The model under review builds one solid part; all positions refer to its coordinate system, in mm. Round coordinates to 2 decimals unless told otherwise and drop trailing zeros. Order: outer loops, then holes, each group sorted by start corner. A loop starts at its lowest first (then second) coordinate and runs counter-clockwise, first axis right, second up. Notation, with made-up numbers: M -39.5,27 L 6.5,27 A16 cw 6.5,41 Z; hole C -3,-35 d7. An arc over 180 degrees is marked long. Answer as a JSON object with one key per item and string values. Group by question number.
1) Consider section B-B, the plane z = 1.8. Count the separate pieces of the cut face and the enclosed holes in it, then the cut area to 3 significant figures.
2) Consider section A-A, the plane x = -129. Write out the cut boundary in (y, z) (3 decimals).
3) To check wall thickness, follow line 1 (X direction, y = 49.5, z = 0.5); line 2 (Y direction, x = -39.5, z = 2.95); line 3 (X direction, y = -125, z = 2.65). State the ranges of each line that lie inside material, in increasing order.
4) Insertion check: pin 1 Ø1.6 at (x, z) = (-99.5, 1) entering from +Y; pin 2 Ø1 at (x, z) = (209, 0.5) entering from -Y; pin 3 Ø7.5 at (x, y) = (-333.55, 0) entering from -Z. Each pin has a flat end and moves straight along its axis. Give the tip position at first contact, or say it passes through.
```python
from build123d import *

# Parameters (mm, degrees)
MASTER_SKETCH_W         = 635.3556
MASTER_SKETCH_H         = 498.348
BOSS_EXTRUDE1_DEPTH     = 3.175
SKETCH2_W               = 31.75
SKETCH2_H               = 498.348
BOSS_EXTRUDE2_DEPTH     = 3.175
M6_CLEARANCE_HOLE1_D    = 6.6
SKETCH5_W               = 2.286
SKETCH5_H               = 69.85
CUT_EXTRUDE1_DEPTH      = 430.182420788
LPATTERN1_COUNT         = 5
LPATTERN1_PITCH         = 98.8568
SKETCH6_W               = 254
SKETCH6_H               = 3.175
CUT_EXTRUDE2_DEPTH      = 430.182420788
SKETCH7_W               = 254
SKETCH7_H               = 2.286
CUT_EXTRUDE3_DEPTH      = 430.182420788
LPATTERN2_COUNT         = 4
LPATTERN2_PITCH         = 98.8568
MIRROR4_COPY_1_SKETCH_W = 254
MIRROR4_COPY_1_SKETCH_H = 2.286
MIRROR4_COPY_1_DEPTH    = 430.182420788
MIRROR4_COPY_2_SKETCH_W = 254
MIRROR4_COPY_2_SKETCH_H = 2.286
MIRROR4_COPY_2_DEPTH    = 430.182420788
MIRROR4_COPY_3_SKETCH_W = 254
MIRROR4_COPY_3_SKETCH_H = 2.286
MIRROR4_COPY_3_DEPTH    = 430.182420788


with BuildPart() as part:
    # Master Sketch → Boss-Extrude1 (new body)
    with BuildSketch(Plane.XY):
        Rectangle(MASTER_SKETCH_W, MASTER_SKETCH_H)
    extrude(amount=BOSS_EXTRUDE1_DEPTH)

    # Sketch2 → Boss-Extrude2 (add)
    with BuildSketch(Plane.XY.offset(3.175)):
        with Locations((-333.5528, 0)):
            Rectangle(SKETCH2_W, SKETCH2_H)
    boss_extrude2 = extrude(amount=-BOSS_EXTRUDE2_DEPTH)

    # M6 Clearance Hole1 (through all)
    with Locations(Plane.XY.offset(3.175)):
        with Locations((-333.5528, -197.612), (-333.5528, -98.806), (-333.5528, 0), (-333.5528, 98.806), (-333.5528, 197.612)):
            m6_clearance_hole1 = Hole(M6_CLEARANCE_HOLE1_D / 2)

    # Mirror1: Boss-Extrude2, M6 Clearance Hole1 across plane
    add(boss_extrude2.mirror(Plane(origin=(0, 0, 0), x_dir=(0, 0, 1), z_dir=(1, 0, 0))))
    add(m6_clearance_hole1.mirror(Plane(origin=(0, 0, 0), x_dir=(0, 0, 1), z_dir=(1, 0, 0))), mode=Mode.SUBTRACT)

    # Sketch5 → Cut-Extrude1 (cut, through all)
    with BuildSketch(Plane.XY.offset(3.175)):
        with Locations((0, 197.7136)):
            Rectangle(SKETCH5_W, SKETCH5_H)
    cut_extrude1 = extrude(amount=-CUT_EXTRUDE1_DEPTH, mode=Mode.SUBTRACT)

    # LPattern1: Cut-Extrude1 ×5
    with Locations(*[(0, -i * LPATTERN1_PITCH, 0) for i in range(1, LPATTERN1_COUNT)]):
        add(cut_extrude1, mode=Mode.SUBTRACT)

    # Sketch6 → Cut-Extrude2 (cut, through all)
    with BuildSketch(Plane.XY.offset(3.175)):
        with Locations((-157.8229, 247.5865)):
            Rectangle(SKETCH6_W, SKETCH6_H)
        with Locations((157.8229, 247.5865)):
            Rectangle(SKETCH6_W, SKETCH6_H)
    cut_extrude2 = extrude(amount=-CUT_EXTRUDE2_DEPTH, mode=Mode.SUBTRACT)

    # Mirror3: Cut-Extrude2 across plane
    add(cut_extrude2.mirror(Plane.ZX), mode=Mode.SUBTRACT)

    # Sketch7 → Cut-Extrude3 (cut, through all)
    with BuildSketch(Plane.XY.offset(3.175)):
        with Locations((-157.8229, 148.2852)):
            Rectangle(SKETCH7_W, SKETCH7_H)
    cut_extrude3 = extrude(amount=-CUT_EXTRUDE3_DEPTH, mode=Mode.SUBTRACT)

    # LPattern2: Cut-Extrude3 ×4
    with Locations(*[(0, -i * LPATTERN2_PITCH, 0) for i in range(1, LPATTERN2_COUNT)]):
        add(cut_extrude3, mode=Mode.SUBTRACT)

    # Mirror4: Cut-Extrude3 across plane
    add(cut_extrude3.mirror(Plane(origin=(0, 0, 0), x_dir=(0, 0, 1), z_dir=(1, 0, 0))), mode=Mode.SUBTRACT)

    # Mirror4 copy 1 sketch → Mirror4 copy 1 (cut, through all)
    with BuildSketch(Plane(origin=(0, -98.8568, 3.175), x_dir=(-1, 0, 0), z_dir=(0, 0, 1))):
        with Locations((-157.8229, -148.2852)):
            Rectangle(MIRROR4_COPY_1_SKETCH_W, MIRROR4_COPY_1_SKETCH_H)
    extrude(amount=-MIRROR4_COPY_1_DEPTH, mode=Mode.SUBTRACT)

    # Mirror4 copy 2 sketch → Mirror4 copy 2 (cut, through all)
    with BuildSketch(Plane(origin=(0, -197.7136, 3.175), x_dir=(-1, 0, 0), z_dir=(0, 0, 1))):
        with Locations((-157.8229, -148.2852)):
            Rectangle(MIRROR4_COPY_2_SKETCH_W, MIRROR4_COPY_2_SKETCH_H)
    extrude(amount=-MIRROR4_COPY_2_DEPTH, mode=Mode.SUBTRACT)

    # Mirror4 copy 3 sketch → Mirror4 copy 3 (cut, through all)
    with BuildSketch(Plane(origin=(0, -296.5704, 3.175), x_dir=(-1, 0, 0), z_dir=(0, 0, 1))):
        with Locations((-157.8229, -148.2852)):
            Rectangle(MIRROR4_COPY_3_SKETCH_W, MIRROR4_COPY_3_SKETCH_H)
    extrude(amount=-MIRROR4_COPY_3_DEPTH, mode=Mode.SUBTRACT)


solid = part.part
```
Results list:
{
 "1": {"separate pieces": "1", "enclosed holes": "23", "area": "339,000 mm^2"},
 "2": {"outline": "M -245.999,0 L -149.428,0 L -149.428,3.175 L -245.999,3.175 Z; M -147.142,0 L -50.571,0 L -50.571,3.175 L -147.142,3.175 Z; M -48.285,0 L 48.285,0 L 48.285,3.175 L -48.285,3.175 Z; M 50.571,0 L 147.142,0 L 147.142,3.175 L 50.571,3.175 Z; M 149.428,0 L 245.999,0 L 245.999,3.175 L 149.428,3.175 Z"},
 "3": {"line 1": "-349.43 to -284.82, -30.82 to 30.82, 284.82 to 349.43", "line 2": "-246 to -149.43, -147.14 to -50.57, -48.29 to 48.29, 50.57 to 147.14, 149.43 to 246", "line 3": "-349.43 to -1.14, 1.14 to 349.43"},
 "4": {"pin 1": "y = 246", "pin 2": "y = -246", "pin 3": "z = 0"}
}
